Geometry check sheet. Reference: the model listing, model coordinates, mm. A direction names the side the tool comes from. Give positions to 0.01 mm unless a question says otherwise; leave off trailing zeros. Write each loop counter-clockwise with the first axis right and the second up, starting at its lowest first coordinate (ties: lowest second). Pieces come first, ordered by that corner, then holes. Notation, with made-up numbers: M 5,-32 L 47,-32 A5 cw 47,-24 Z; hole C 57,80 d5. An arc over 180 degrees is marked long. One line per item, written item: value. Start each with the question number.
1. Gauge pin test, flat ends, axial feed: pin 1 (1 mm diameter, centred on x = 3.5, z = 6.5, fed in from -Y); pin 2 (3.5 mm diameter, centred on x = 0, z = 6.14, fed in from -Y); pin 3 (1.5 mm diameter, centred on y = -33, z = 18, fed in from -X). Record the tip position at first contact, or that the pin passes through.
2. Release check for a two-part mould opening along Z. For faces 4 (the face through (-12.474, -86.204, 14.804)), 5 (the face through (25, -5, 15)), 6 (the face through (0, -15, 15)) record: pulls with the +Z half, pulls with the -Z half, needs draft (parallel to the pull), parting line crosses it, or undercut.
3. Scan lines: line 1 (Z direction, x = 0, y = -69); line 2 (Z direction, x = 20, y = -8); line 3 (X direction, y = -24, z = 18.25). Record each from-to range of solid material in increasing order.
4. Cross-section at C-C on x = 4. Record the cut outline in (y, z) (3 decimals), then the cut area to 3 significant figures.
5. Cross-section at A-A on z = 14.75. Count the separate pieces of the cut face and the enclosed holes in it, then the cut area to 3 significant figures.
6. Cross-section at B-B on x = 20. Record the cut outline in (y, z).
7. Tool access check on faces 1 (the face through (20, -69, 15)), 2 (the face through (17.9, -7.8, 14.7)), 3 (the face through (-20, -69, 15)). Record the directions out of +Z, -Z, +X, -X, +Y, -Y that give a thin tool (end or side, any length) a straight path to the whole face; none if there is none.
8. Cross-section at D-D on y = -56.5. Record the cut outline in (x, z), then the cut area to 3 significant figures.
from build123d import *

# Parameters (mm, degrees)
BOSS_EXTRUDE1_DEPTH = 29.5
BOSS_EXTRUDE2_DEPTH = 7
CHAMFER1_SIZE       = 0.5
M5X0_82_D           = 4.2
M5X0_82_DEPTH       = 19
M5X0_82_TIP         = 1.2618073
SKETCH13_W          = 8.675232358
SKETCH13_H          = 9.5
M5X0_81_REACH       = 99.955
M5X0_81_BORE_R      = 2.1
CHAMFER_1_SIZE      = 1


with BuildPart() as part:
    # Sketch1 → Boss-Extrude1 (new body)
    with BuildSketch(Plane.XY):
        with BuildLine():
            Line((12, 0), (25, 0))
            Line((25, 0), (25, -10))
            Line((25, -10), (15, -18))
            Line((15, -18), (15, -65))
            Line((15, -65), (25, -73))
            Line((25, -73), (25, -83))
            Line((25, -83), (-25, -83))
            Line((-25, -83), (-25, -73))
            Line((-25, -73), (-15, -65))
            Line((-15, -65), (-15, -18))
            Line((-15, -18), (-25, -10))
            Line((-25, -10), (-25, 0))
            Line((-25, 0), (-12, 0))
            ThreePointArc((-12, 0), (0, -12), (12, 0))
        make_face()
    extrude(amount=BOSS_EXTRUDE1_DEPTH)

    # Sketch2 → Boss-Extrude2 (add)
    with BuildSketch(Plane.XZ.offset(83)):
        with BuildLine():
            Line((-10, 12.275), (10, 12.275))
            ThreePointArc((10, 12.275), (12.475, 14.75), (10, 17.225))
            Line((10, 17.225), (-10, 17.225))
            ThreePointArc((-10, 17.225), (-12.475, 14.75), (-10, 12.275))
        make_face()
    extrude(amount=BOSS_EXTRUDE2_DEPTH)

    # Chamfer1
    chamfer1_edges = [part.edges().sort_by_distance(p)[0] for p in [
        (12.475, -90, 14.75),
        (0, -90, 17.225),
        (-12.475, -90, 14.75),
        (0, -90, 12.275),
    ]]
    chamfer(chamfer1_edges, length=CHAMFER1_SIZE)

    # Отверстие обработанное метчиком M5x0.82
    with Locations(Plane(origin=(0, -83, 0), x_dir=(-1, 0, 0), z_dir=(0, -1, 0))):
        with Locations((0, -23.3625), (0, -6.1375)):
            Hole(M5X0_82_D / 2, depth=M5X0_82_DEPTH)
            with Locations((0, 0, -(M5X0_82_DEPTH + M5X0_82_TIP / 2))):  # 118° drill point
                Cone(0, M5X0_82_D / 2, M5X0_82_TIP, mode=Mode.SUBTRACT)

    # Sketch13 → Cut-Revolve1 (revolve, cut)
    with BuildSketch(Plane(origin=(0, 0, 0), x_dir=(1, 0, 0), z_dir=(0, 1, 0))):
        with Locations((-10.662383821, -14.75)):
            Rectangle(SKETCH13_W, SKETCH13_H)
    revolve(axis=Axis((0, 0, 0), (0, 0, 1)), mode=Mode.SUBTRACT)

    # Отверстие обработанное метчиком M5x0.81 bore → Отверстие обработанное метчиком M5x0.81 (cut, up to next)
    with BuildSketch(Plane(origin=(0, 0, 0), x_dir=(1, 0, 0), z_dir=(0, 1, 0)), mode=Mode.PRIVATE) as m5x0_81_sk1:
        with Locations((-20, -14.75)):
            Circle(M5X0_81_BORE_R)
    m5x0_81_tool1 = extrude(m5x0_81_sk1.sketch, amount=-M5X0_81_REACH, mode=Mode.PRIVATE) & part.part
    # Отверстие обработанное метчиком M5x0.81 bore → Отверстие обработанное метчиком M5x0.81 (cut, up to next)
    with BuildSketch(Plane(origin=(0, 0, 0), x_dir=(1, 0, 0), z_dir=(0, 1, 0)), mode=Mode.PRIVATE) as m5x0_81_sk2:
        with Locations((20, -14.75)):
            Circle(M5X0_81_BORE_R)
    m5x0_81_tool2 = extrude(m5x0_81_sk2.sketch, amount=-M5X0_81_REACH, mode=Mode.PRIVATE) & part.part
    add(m5x0_81_tool1.solids().sort_by_distance((-20, 0, 14.75))[0], mode=Mode.SUBTRACT)
    add(m5x0_81_tool2.solids().sort_by_distance((20, 0, 14.75))[0], mode=Mode.SUBTRACT)

    # Фаска1
    chamfer_1_edges = [part.edges().sort_by_distance(p)[0] for p in [
        (-25, 0, 14.75),
        (25, 0, 14.75),
    ]]
    chamfer(chamfer_1_edges, length=CHAMFER_1_SIZE)


solid = part.part
Report:
1. pin 1: stops at y = -83
1. pin 2: stops at y = -63.79
1. pin 3: stops at x = -15
2. face 4: parting line crosses it
2. face 5: needs draft
2. face 6: undercut
3. line 1: z = 0 to 4.04, 8.24 to 21.26, 25.46 to 29.5
3. line 2: z = 0 to 12.65, 16.85 to 29.5
3. line 3: x = -15 to 15
4. outline: M -90,12.775 L -89.5,12.275 L -83,12.275 L -83,0 L -11.314,0 L -11.314,10 L -14.457,10 L -14.457,19.5 L -11.314,19.5 L -11.314,29.5 L -83,29.5 L -83,17.225 L -89.5,17.225 L -90,16.725 Z
4. area: 2,120 mm^2
5. separate pieces: 3
5. enclosed holes: 0
5. area: 2,750 mm^2
6. outline: M -83,0 L -69,0 L -69,29.5 L -83,29.5 Z; M -14,0 L 0,0 L 0,12.65 L -14,12.65 Z; M -14,16.85 L 0,16.85 L 0,29.5 L -14,29.5 Z
7. face 1: +Z, -Z, +X
7. face 2: +Y
7. face 3: +Z, -Z, -X
8. outline: M -15,0 L 15,0 L 15,29.5 L -15,29.5 Z
8. area: 885 mm^2
